```python
from build123d import *

# Parameters (mm, degrees)
F0_R     = 1.625
F1_DEPTH = 5
F2_R     = 3.05
F3_DEPTH = 3.5
F4_W     = 4.79
F4_H     = 2.71
F5_DEPTH = 43.45


with BuildPart() as f1:
    # F0 (on Top) → F1 (new body)
    with BuildSketch(Plane.XY):
        with BuildLine():
            Line((22.5, 25), (-32.5, 25))
            ThreePointArc((-32.5, 25), (-36.035534, 23.535534), (-37.5, 20))
            Line((-37.5, 20), (-37.5, -30))
            ThreePointArc((-37.5, -30), (-36.035534, -33.535534), (-32.5, -35))
            ThreePointArc((-32.5, -35), (-28.964466, -33.535534), (-27.5, -30))
            ThreePointArc((-27.5, -30), (-26.035534, -26.464466), (-22.5, -25))
            Line((-22.5, -25), (22.5, -25))
            ThreePointArc((22.5, -25), (26.035534, -23.535534), (27.5, -20))
            Line((27.5, -20), (27.5, 20))
            ThreePointArc((27.5, 20), (26.035534, 23.535534), (22.5, 25))
        make_face()
        with Locations((-32.5, -30)):
            Circle(F0_R, mode=Mode.SUBTRACT)
        with Locations((17.4, -10)):
            Circle(F0_R, mode=Mode.SUBTRACT)
        with Locations((17.4, 10)):
            Circle(F0_R, mode=Mode.SUBTRACT)
    extrude(amount=F1_DEPTH)

    # F2 (on face) → F3 (cut)
    with BuildSketch(Plane.XY.offset(5)):
        with Locations((17.4, 10)):
            Circle(F2_R)
        with Locations((17.4, -10)):
            Circle(F2_R)
        with Locations((-32.5, -30)):
            Circle(F2_R)
    extrude(amount=-F3_DEPTH, mode=Mode.SUBTRACT)

    # F4 (on face) → F5 (cut, symmetric)
    with BuildSketch(Plane.XZ.offset(25)):
        with Locations((-20.105, 1.355)):
            Rectangle(F4_W, F4_H)
        Polygon((4.7, 2.71), (4.7, 0), (12.88, 0), (14.29, 2.71), align=None)
        Polygon((-25.89, 0), (-22.5, 0), (-22.5, 2.71), (-27.3, 2.71), align=None)
    extrude(amount=F5_DEPTH, both=True, mode=Mode.SUBTRACT)


solid = f1.part
```
Check sheet for the modelled part. Datum: model origin and axes. Units: mm. A direction names the side the tool comes from. Coordinates: 2 decimals unless noted, no trailing zeros. Loops run counter-clockwise (first coordinate to the right, second up) from the corner with the lowest first, then second, coordinate; pieces in that order, holes last. Notation, with made-up numbers: M 20,84 L 64,84 A21 cw 64,99 Z; hole C 48,56 d4. An arc over 180 degrees is marked long. Answer as a JSON object with one key per item and string values.
1. Depth check by flat-ended pin: P1, Ø3, axis at x = -23.5, y = -2.5, coming from the -Z side; P2, Ø1.5, axis at x = 3.5, z = 2, coming from the -Y side; P3, Ø1.4, axis at x = -24.5, z = 1.5, coming from the -Y side. Enter the tip coordinate at first touch or a pass-through.
Outcome:
{"P1": "z = 2.71", "P2": "y = -25", "P3": "y = 18.45"}
2. Sectioned sample at B-B on x = 17.4. Record the cut outline in (y, z) (3 decimals), and give its area (3 significant figures).
Outcome:
{"outline": "M -25,0 L -11.625,0 L -11.625,1.5 L -13.05,1.5 L -13.05,5 L -25,5 Z; M -8.375,0 L 8.375,0 L 8.375,1.5 L 6.95,1.5 L 6.95,5 L -6.95,5 L -6.95,1.5 L -8.375,1.5 Z; M 11.625,0 L 25,0 L 25,5 L 13.05,5 L 13.05,1.5 L 11.625,1.5 Z", "area": "198 mm²"}
3. Release check for a two-part mould opening along Y. For faces 1 (the cylindrical face through (26, -23.57, 2.46)), 2 (the flat face through (-37.5, -5, 2)), 3 (the cylindrical face through (17.19, -8.39, 0.74)) record: pulls with the +Y half, pulls with the -Y half, needs draft (parallel to the pull), parting line crosses it, or undercut.
Outcome:
{"face 1": "pulls with the -Y half", "face 2": "needs draft", "face 3": "undercut"}
4. Sectioned sample at A-A on y = 10. Record the cut outline in (x, z) (3 decimals), and give its area (3 significant figures).
Outcome:
{"outline": "M -37.5,0 L -25.89,0 L -27.3,2.71 L -17.71,2.71 L -17.71,0 L 4.7,0 L 4.7,2.71 L 14.29,2.71 L 12.88,0 L 15.775,0 L 15.775,1.5 L 14.35,1.5 L 14.35,5 L -37.5,5 Z; M 19.025,0 L 27.5,0 L 27.5,5 L 20.45,5 L 20.45,1.5 L 19.025,1.5 Z", "area": "251 mm²"}
5. Sectioned sample at D-D on y = 1.5. Record the cut outline in (x, z), and give its area (3 significant figures).
Outcome:
{"outline": "M -37.5,0 L -25.89,0 L -27.3,2.71 L -17.71,2.71 L -17.71,0 L 4.7,0 L 4.7,2.71 L 14.29,2.71 L 12.88,0 L 27.5,0 L 27.5,5 L -37.5,5 Z", "area": "277 mm²"}
6. Sectioned sample at C-C on x = -18.5. Record the cut outline in (y, z), and give its area (3 significant figures).
Outcome:
{"outline": "M -25,2.71 L 18.45,2.71 L 18.45,0 L 25,0 L 25,5 L -25,5 Z", "area": "132 mm²"}
7. Scan lines: L1, parallel to Y at x = 17.4, z = 0.5 (3 decimals); L2, parallel to Y at x = 17.4, z = 2.4; L3, parallel to X at y = -10, z = 0.95 (3 decimals). Record each from-to range of solid material in increasing order. Write a range as from..to.
Outcome:
{"L1": "-25..-11.625, -8.375..8.375, 11.625..25", "L2": "-25..-13.05, -6.95..6.95, 13.05..25", "L3": "-37.5..-26.384, -17.71..4.7, 13.374..15.775, 19.025..27.5"}
8. Access from +Z, -Z, +X, -X, +Y, -Y to the whole of each face (thin tool, end or side, straight path). Record for faces 4 (the flat face through (13.575, -3.579, 1.336)), 5 (the flat face through (-31, -31, 1.5)), 6 (the flat face through (4.7, -4, 1)).
Outcome:
{"face 4": "-Y", "face 5": "+Z", "face 6": "-Z, -Y"}
